```python
from build123d import *

# Parameters (mm, degrees)
F0_W        = 35
F0_H        = 2
F1_DEPTH    = 25
F2_T1_DEPTH = 33.357808199
F3_R        = 2


# Not quite as in the source:
# - a fillet or chamfer that OpenCascade refuses, or shapes differently, is made with other operations: its cross-section is extruded or revolved along the edge and cut away or added


with BuildPart() as f1:
    # F0 (on Top) → F1 (new body)
    with BuildSketch(Plane.XY):
        with Locations((0, 17)):
            Rectangle(F0_W, F0_H)
        with BuildLine():
            ThreePointArc((-5.6435050377, 2.0373637106), (0, 6), (5.6435050377, 2.0373637106))
            add(Edge.make_bspline(
                [(17.5, 16), (-4.7855940647, 13.2096234411), (3.9503478981, 6.7274152696), (5.6435050377, 2.0373637106)],
                knots=[0, 0, 0, 0, 18.317523985, 18.317523985, 18.317523985, 18.317523985], degree=3))
            Line((17.5, 16), (-17.5, 16))
            add(Edge.make_bspline(
                [(-17.5, 16), (4.7855940647, 13.2096234411), (-3.9503478981, 6.7274152696), (-5.6435050377, 2.0373637106)],
                knots=[0, 0, 0, 0, 18.317523985, 18.317523985, 18.317523985, 18.317523985], degree=3))
        make_face()
        with BuildLine():
            ThreePointArc((-1.5493444278, -4.7538964907), (0, 5), (1.5493444278, -4.7538964907))
            Line((1.5493444278, -4.7538964907), (1.5493444278, -5.7965103161))
            ThreePointArc((1.5493444278, -5.7965103161), (3.7756538243, -4.6630932007), (5.3474024613, -2.7212656829))
            ThreePointArc((5.3474024613, -2.7212656829), (5.9884180164, -0.3726253627), (5.6435050377, 2.0373637106))
            ThreePointArc((5.6435050377, 2.0373637106), (0, 6), (-5.6435050377, 2.0373637106))
            ThreePointArc((-5.6435050377, 2.0373637106), (-5.9884180164, -0.3726253627), (-5.3474024613, -2.7212656829))
            ThreePointArc((-5.3474024613, -2.7212656829), (-3.7756538243, -4.6630932007), (-1.5493444278, -5.7965103161))
            Line((-1.5493444278, -5.7965103161), (-1.5493444278, -4.7538964907))
        make_face()
        with BuildLine():
            Line((-2.6496251192, -7.5926648612), (-1.5493444278, -5.7965103161))
            ThreePointArc((-1.5493444278, -5.7965103161), (-3.7756538243, -4.6630932007), (-5.3474024613, -2.7212656829))
            add(Edge.make_bspline(
                [(-5.3474024613, -2.7212656829), (-4.3048003044, -4.7700231324), (-2.8869232094, -5.6816728311), (-3.8415154138, -6.828782889)],
                knots=[0, 0, 0, 0, 4.2754829053, 4.2754829053, 4.2754829053, 4.2754829053], degree=3))
            ThreePointArc((-3.8415154138, -6.828782889), (-3.8851139698, -6.989281561), (-3.7922551547, -7.1272594514))
            Line((-3.7922551547, -7.1272594514), (-2.9246420572, -7.6587381827))
            ThreePointArc((-2.9246420572, -7.6587381827), (-2.7734493553, -7.6826593947), (-2.6496251192, -7.5926648612))
        make_face()
        with BuildLine():
            ThreePointArc((5.3474024613, -2.7212656829), (3.7756538243, -4.6630932007), (1.5493444278, -5.7965103161))
            Line((1.5493444278, -5.7965103161), (2.6496251192, -7.5926648612))
            ThreePointArc((2.6496251192, -7.5926648612), (2.7734493553, -7.6826593947), (2.9246420572, -7.6587381827))
            Line((2.9246420572, -7.6587381827), (3.7922551547, -7.1272594514))
            ThreePointArc((3.7922551547, -7.1272594514), (3.8851139698, -6.989281561), (3.8415154138, -6.828782889))
            add(Edge.make_bspline(
                [(5.3474024613, -2.7212656829), (4.3048003044, -4.7700231324), (2.8869232094, -5.6816728311), (3.8415154138, -6.828782889)],
                knots=[0, 0, 0, 0, 4.2754829053, 4.2754829053, 4.2754829053, 4.2754829053], degree=3))
        make_face()
    extrude(amount=F1_DEPTH)

    # F2: fillet of radius 5 on 2 edges, made by hand

    # F2_s2 → F2_t1 (cut)
    with BuildSketch(Plane.XY.offset(-4.1789040995)):
        with BuildLine():
            ThreePointArc((-1.5493444278, -5.7965103161), (-2.1813631769, -4.7990149212), (-3.0296890274, -3.9775601061))
            ThreePointArc((-3.0296890274, -3.9775601061), (-2.3221889224, -4.4280287498), (-1.5493444278, -4.7538964907))
            Line((-1.5493444278, -4.7538964907), (-1.5493444278, -5.7965103161))
        make_face()
        with BuildLine():
            ThreePointArc((3.0296890274, -3.9775601061), (2.1813631769, -4.7990149212), (1.5493444278, -5.7965103161))
            Line((1.5493444278, -5.7965103161), (1.5493444278, -4.7538964907))
            ThreePointArc((1.5493444278, -4.7538964907), (2.3221889224, -4.4280287498), (3.0296890274, -3.9775601061))
        make_face()
    extrude(amount=F2_T1_DEPTH, mode=Mode.SUBTRACT)

    # F3
    f3_edges = [f1.edges().sort_by_distance(p)[0] for p in [
        (-1.549344, -5.79651, 12.5),
        (1.549344, -5.79651, 12.5),
    ]]
    fillet(f3_edges, radius=F3_R)


solid = f1.part
```
CAD build for the part. Positions are in the model's coordinates, mm. A direction names the side the tool comes from. Round coordinates to 2 decimals unless told otherwise and drop trailing zeros. Order: outer loops, then holes, each group sorted by start corner. A loop starts at its lowest first (then second) coordinate and runs counter-clockwise, first axis right, second up. Notation, with made-up numbers: (83, 19.25) - (111, 19.25) arc R26 cw to (111, 45.25) - close; hole circle Ø7 at (14.5, -5). An arc over 180 degrees is marked (long way). Use CSV: the item, a comma, the result in double quotes. Start each with the question number.
1) Two-plate mould, pull along Y, no slides. Class faces 1 (the flat face through (0, 12, 25)), 2 (the flat face through (-3.36, -7.39, 12.32)), 3 (the cylindrical face through (1.937, -5.636, 12.675)): pulls with the +Y half, pulls with the -Y half, needs draft (parallel to the pull), parting line crosses it, or undercut.
2) Pin check, flat tips, straight feed: pin 1 Ø2 at (y, z) = (-2, 5.5) entering from -X; pin 2 Ø8 at (y, z) = (-4, 19) entering from +X; pin 3 Ø8 at (x, y) = (0, 0) entering from -Z. Stop position of each tip, or through.
3) Saw through at B-B (x = 0). List the corners of the cut face in (y, z).
4) Tool access for faces 4 (the cylindrical face through (-1.94, -5.6, 12.68)), 5 (the flat face through (0, 18, 12)): list every direction of +Z, -Z, +X, -X, +Y, -Y with a clear straight run to the whole face (end or side of a thin tool).
5) Saw through at A-A (y = 0). List the corners of the cut face in (x, z).
6) Wall check: L1, parallel to X at y = 0, z = 14; L2, parallel to Y at x = 0, z = 9.75; L3, parallel to X at y = 9, z = 17.25. Give the ranges that are in metal, low to high. Write a range as [from, to].
Values follow:
1,face 1,"needs draft"
1,face 2,"pulls with the -Y half"
1,face 3,"undercut"
2,pin 1,"stops at x = -5.92"
2,pin 2,"stops at x = 6"
2,pin 3,"passes through"
3,outline,"(5, 0) - (18, 0) - (18, 25) - (5, 25) - close"
4,face 4,"+Z, -Z"
4,face 5,"+Z, -Z, +X, -X, +Y"
5,outline,"(-6, 0) - (-5, 0) - (-5, 25) - (-6, 25) - close; (5, 0) - (6, 0) - (6, 25) - (5, 25) - close"
6,L1,"x = [-6, -5], [5, 6]"
6,L2,"y = [5, 18]"
6,L3,"x = [-2.55, 2.55]"
